Can you work these out from the drawing? Everything is in mm from the part's minimum corner. A direction names the side the tool comes from. Round coordinates to 2 decimals unless told otherwise and drop trailing zeros. Order: outer loops, then holes, each group sorted by start corner. A loop starts at its lowest first (then second) coordinate and runs counter-clockwise, first axis right, second up. Notation, with made-up numbers: M -16,29.5 L 6,29.5 A14 cw 6,54.5 Z; hole C 81.5,35 d8. An arc over 180 degrees is marked long. Write each question's results on one line, items separated by ' | '. Start each with the question number.
1. We'd pull the mould along X, two halves only. Please class the marked faces 1, 2, 3 and 4: released by +X, released by -X, zero draft, split by the parting line, or undercut.
2. Suppose I cut it at B-B on z = 41.5. Write out the boundary of the cut face in (x, y).
3. I'm going to push flat-ended pins straight in: pin 1 (6 mm diameter, centred on y = 10, z = 14.5, fed in from -X); pin 2 (2 mm diameter, centred on x = 3.5, y = 6, fed in from -Z); pin 3 (8 mm diameter, centred on x = 11, y = 15.5, fed in from -Z); pin 4 (5 mm diameter, centred on x = 24.5, y = 20, fed in from -Z). Where does each tip first touch, or does it pass through?
4. Suppose I cut it at D-D on x = 11. Write out the boundary of the cut face in (y, z), and give its area (3 significant figures).
5. Please list where these lines run through material, in increasing order: L1, parallel to X at y = 16, z = 12.5; L2, parallel to Z at x = 11, y = 10.5; L3, parallel to Z at x = 26, y = 11.25.
6. For the marked faces 5, 6 and 7, which set-ups out of +Z, -Z, +X, -X, +Y, -Y let a thin tool reach every point of the face, with its end or its side?
7. Suppose I cut it at A-A on z = 14.5. Write out the boundary of the cut face in (x, y).
8. Suppose I cut it at C-C on y = 19.25. Write out the boundary of the cut face in (x, z).
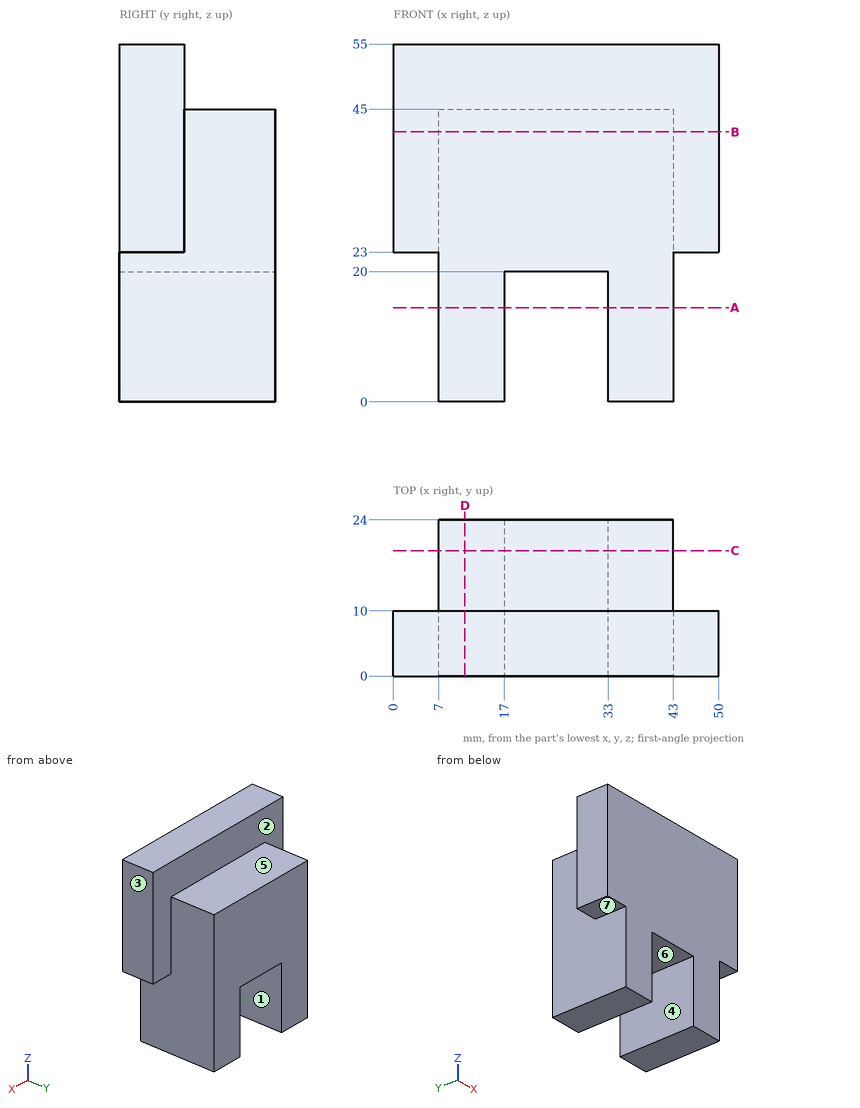
Filled sheet:
1) face 1: undercut | face 2: zero draft | face 3: released by +X | face 4: undercut
2) outline: M 0,0 L 50,0 L 50,10 L 43,10 L 43,24 L 7,24 L 7,10 L 0,10 Z
3) pin 1: stops at x = 7 | pin 2: stops at z = 23 | pin 3: stops at z = 0 | pin 4: stops at z = 20
4) outline: M 0,0 L 24,0 L 24,45 L 10,45 L 10,55 L 0,55 Z | area: 1,180 mm^2
5) L1: x = 7 to 17, 33 to 43 | L2: z = 0 to 45 | L3: z = 20 to 45
6) face 5: +Z, +X, -X, +Y | face 6: -Z, +Y, -Y | face 7: -Z, -X, +Y, -Y
7) outline: M 7,0 L 17,0 L 17,24 L 7,24 Z; M 33,0 L 43,0 L 43,24 L 33,24 Z
8) outline: M 7,0 L 17,0 L 17,20 L 33,20 L 33,0 L 43,0 L 43,45 L 7,45 Z
